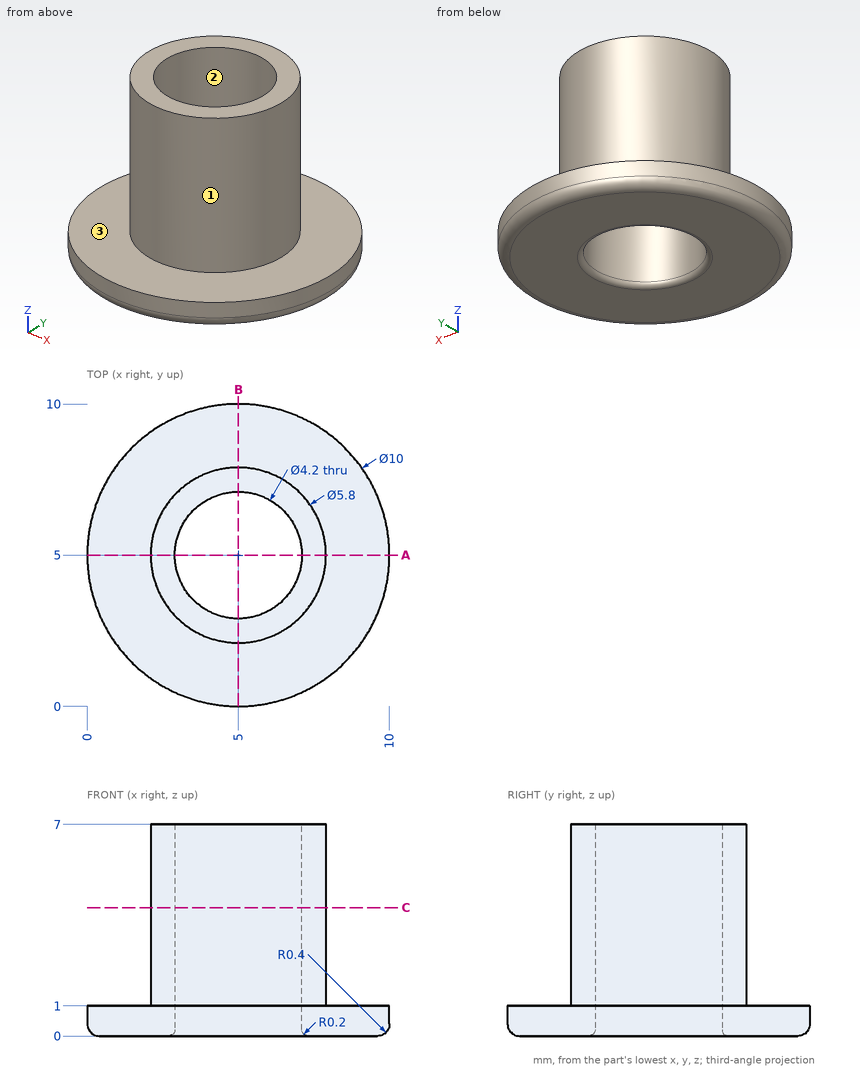
For this review, use the dimensioned drawing (mm, ordinates from the lowest corner) and the shaded views. Round coordinates to 2 decimals unless told otherwise and drop trailing zeros. Order: outer loops, then holes, each group sorted by start corner. A loop starts at its lowest first (then second) coordinate and runs counter-clockwise, first axis right, second up.
1) Clearance check with flat-ended pins moving along their axes: pin 1 Ø4 at (x, z) = (7.5, 1.5) entering from -Y; pin 2 Ø1 at (y, z) = (4, 3.5) entering from +X; pin 3 Ø2.5 at (x, y) = (5, 5) entering from +Z. State where each tip first meets the part, or that it passes through.
The answers:
pin 1: stops at y = 0.03
pin 2: stops at x = 7.86
pin 3: passes through
2) Consider section A-A (y = 5). State the section outline as (x, z) points.
The answers:
outline: (0, 0.4) arc R0.4 ccw to (0.4, 0) - (2.7, 0) arc R0.2 ccw to (2.9, 0.2) - (2.9, 7) - (2.1, 7) - (2.1, 1) - (0, 1) - close; (7.1, 0.2) arc R0.2 ccw to (7.3, 0) - (9.6, 0) arc R0.4 ccw to (10, 0.4) - (10, 1) - (7.9, 1) - (7.9, 7) - (7.1, 7) - close
3) Consider section C-C (z = 4.25). State the section outline as (x, y) points.
The answers:
outline: circle Ø5.8 at (5, 5); hole circle Ø4.2 at (5, 5)
4) Draft analysis for pull direction Y (two halves, no side actions). For the marked faces 1, 2 and 3, state which applies: released by +Y, released by -Y, zero draft, split by the parting line, or undercut.
The answers:
face 1: split by the parting line
face 2: undercut
face 3: zero draft
5) For L1, parallel to Y at x = 5, z = 4.75; L2, parallel to Z at x = 1.5, y = 6; L3, parallel to X at y = 6, z = 4, list the stretches that pass through material, from the lowest coordinate up.
The answers:
L1: y = 2.1 to 2.9, 7.1 to 7.9
L2: z = 0 to 1
L3: x = 2.28 to 3.15, 6.85 to 7.72
